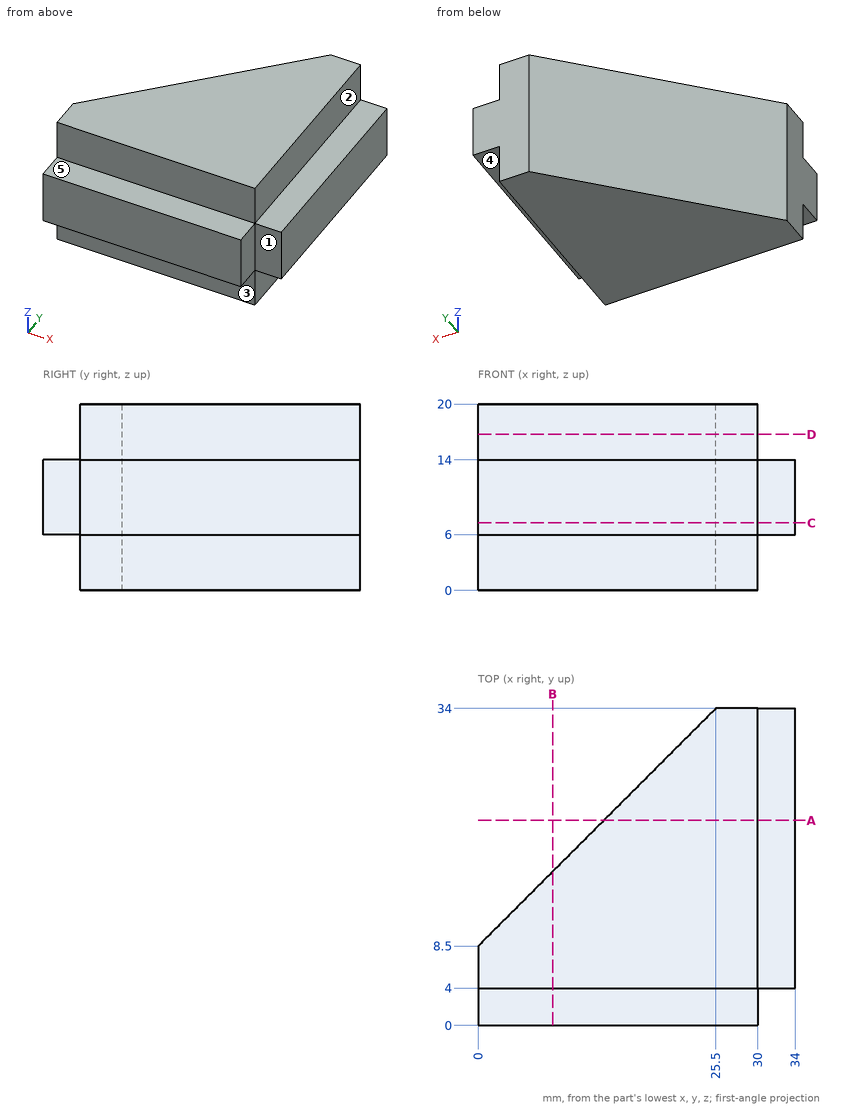
Check sheet for the drawn part. Datum: minimum x, y, z corner. Units: mm. A direction names the side the tool comes from. Round coordinates to 2 decimals unless told otherwise and drop trailing zeros. Order: outer loops, then holes, each group sorted by start corner. A loop starts at its lowest first (then second) coordinate and runs counter-clockwise, first axis right, second up.
1. Section check D-D on z = 16.75. Record the cut outline in (x, y).
Final values:
outline: (0, 4) - (30, 4) - (30, 34) - (25.5, 34) - (0, 8.5) - close
2. Thickness scan on L1, parallel to Y at x = 17, z = 12.25; L2, parallel to Z at x = 32, y = 14.5; L3, parallel to Y at x = 5.5, z = 2.25. Record the ranges inside material, lowest first.
Final values:
L1: y = 0 to 25.5
L2: z = 6 to 14
L3: y = 4 to 14
3. Access from +Z, -Z, +X, -X, +Y, -Y to the whole of each face (thin tool, end or side, straight path). Record for the marked faces 1, 2, 3, 4 and 5.
Final values:
face 1: +Z, -Z, +X, -Y
face 2: +Z, +X, +Y, -Y
face 3: -Z, +X, -X, -Y
face 4: -Z, +X, +Y, -Y
face 5: +Z, +X, -X, -Y
4. Section check B-B on x = 8. Record the cut outline in (y, z).
Final values:
outline: (0, 6) - (4, 6) - (4, 0) - (16.5, 0) - (16.5, 20) - (4, 20) - (4, 14) - (0, 14) - close
5. Go/stop test with flat-tipped pins: P1, Ø6.5, axis at y = 15, z = 16.5, coming from the +X side; P2, Ø4.5, axis at x = 33, y = 20, coming from the -Z side; P3, Ø8, axis at x = 10.5, z = 18, coming from the +Y side; P4, Ø1.2, axis at x = 8, y = 2, coming from the +Z side. Record where each tip stops, or that it passes through.
Final values:
P1: stops at x = 34
P2: stops at z = 6
P3: stops at y = 23
P4: stops at z = 14
6. Section check A-A on y = 22. Record the cut outline in (x, z), then the cut area to 3 significant figures.
Final values:
outline: (13.5, 0) - (30, 0) - (30, 6) - (34, 6) - (34, 14) - (30, 14) - (30, 20) - (13.5, 20) - close
area: 362 mm2
7. Section check C-C on z = 7.25. Record the cut outline in (x, y).
Final values:
outline: (0, 0) - (30, 0) - (30, 4) - (34, 4) - (34, 34) - (25.5, 34) - (0, 8.5) - close
